The listing builds one solid part. Answer for the finished solid, in the listing's coordinates (mm). A direction names the side the tool comes from. Coordinates: 2 decimals unless noted, no trailing zeros. Write each loop counter-clockwise with the first axis right and the second up, starting at its lowest first coordinate (ties: lowest second). Pieces come first, ordered by that corner, then holes. Notation, with made-up numbers: M 42,50.25 L 58,50.25 A25 cw 58,65.25 Z; hole C 69,54 d8. An arc over 180 degrees is marked long. Answer as CSV lines item,"result". Start each with the question number.
```python
from build123d import *

# Parameters (mm, degrees)
EXTRUDE_1_DEPTH      = 90
EXTRUDE_3_DEPTH      = 45
EXTRUDE_3_DEPTH_BACK = 45
SKETCH_2_R           = 10


with BuildPart() as part:
    # Эскиз1 → Вытянуть-Тонкостенный1 (new body)
    with BuildSketch(Plane.XY):
        with BuildLine():
            Line((60, 20), (0, 20))
            ThreePointArc((0, 20), (-20, 0), (0, -20))
            Line((0, -20), (60, -20))
            Line((60, -20), (60, -10))
            Line((60, -10), (0, -10))
            ThreePointArc((0, -10), (-10, 0), (0, 10))
            Line((0, 10), (60, 10))
            Line((60, 10), (60, 20))
        make_face()
    extrude(amount=EXTRUDE_1_DEPTH)

    # Эскиз2 → Бобышка-Вытянуть3 (add, two sides: drawn at the far end of the back side and taken through both)
    with BuildSketch(Plane(origin=(0, 0, 0), x_dir=(1, 0, 0), z_dir=(0, 1, 0)).offset(-EXTRUDE_3_DEPTH_BACK)):
        with BuildLine():
            Line((-20, -25), (-20, -65))
            Line((-20, -65), (40, -65))
            ThreePointArc((40, -65), (59.396542923, -45), (40, -25))
            Line((40, -25), (-20, -25))
        make_face()
        with Locations(Location((39.387155672, -45, 0), (0, 0, 270))):
            Circle(SKETCH_2_R, mode=Mode.SUBTRACT)
    extrude(amount=EXTRUDE_3_DEPTH + EXTRUDE_3_DEPTH_BACK)


solid = part.part
```
1) The part is cut by section B-B (x = 3). Determine the outline of the cut face in (y, z), then the cut area to 3 significant figures.
2) Each of these flat-tipped pins is pushed along its axis until it touches: P1, Ø16, axis at x = 43, z = 43.5, coming from the -Y side; P2, Ø18, axis at x = 39.39, z = 45, coming from the -Y side; P3, Ø18, axis at x = 39.39, z = 45, coming from the +Y side; P4, Ø2, axis at x = 2.5, y = -24.5, coming from the +Z side. Where does it stop, or does it pass through?
3) For a pull along Z with two mould halves and no side action, classify faces 4 (the face through (39.83, -0.14, 35.01)), 5 (the face through (59.39, -32.67, 45.43)), 6 (the face through (-20, 0, 12)) as +Z half, -Z half, draft (parallel to the pull), parting line (faces both ways), or undercut.
4) Find the intervals of material crossed by line 1 (X direction, y = 35, z = 45); line 2 (Y direction, x = 23, z = 81); line 3 (Z direction, x = 10, y = 7.5), in increasing order. Write a range as from..to.
5) Which of the six approach directions +Z, -Z, +X, -X, +Y, -Y give full straight-line access (tool end or side, diameter ignored) to faces 1 (the face through (39, 10, 45)), 2 (the face through (-10, 0, 12)), 3 (the face through (30, 10, 24))?
6) The part is cut by section D-D (z = 17.5). Determine the outline of the cut face in (x, y), then the cut area to 3 significant figures.
7) The part is cut by section A-A (z = 45). Determine the outline of the cut face in (x, y), then the cut area to 3 significant figures.
8) The part is cut by section C-C (y = -3.5). Determine the outline of the cut face in (x, z).
Completed:
1,outline,"M -45,25 L -20,25 L -20,0 L -10,0 L -10,25 L 10,25 L 10,0 L 20,0 L 20,25 L 45,25 L 45,65 L 20,65 L 20,90 L 10,90 L 10,65 L -10,65 L -10,90 L -20,90 L -20,65 L -45,65 Z"
1,area,"4,600 mm²"
2,P1,"y = -45"
2,P2,"y = -20"
2,P3,"y = 20"
2,P4,"z = 65"
3,face 4,"undercut"
3,face 5,"parting line"
3,face 6,"draft"
4,line 1,"-20..29.39, 49.39..59.4"
4,line 2,"-20..-10, 10..20"
4,line 3,"25..65"
5,face 1,"none"
5,face 2,"-Z, +X"
5,face 3,"+X"
6,outline,"M 0,-20 L 60,-20 L 60,-10 L 0,-10 A10 cw 0,10 L 60,10 L 60,20 L 0,20 A20 ccw Z"
6,area,"1,670 mm²"
7,outline,"M -20,-45 L 29.39,-45 L 29.39,-20 L 49.39,-20 L 49.39,-45 L 59.4,-45 L 59.4,-20 L 60,-20 L 60,-10 L 59.4,-10 L 59.4,10 L 60,10 L 60,20 L 59.4,20 L 59.4,45 L 49.39,45 L 49.39,20 L 29.39,20 L 29.39,45 L -20,45 Z; hole M 29.39,-10 L 49.39,-10 L 49.39,10 L 29.39,10 Z"
7,area,"5,760 mm²"
8,outline,"M -20,25 L -19.69,25 L -19.69,0 L -9.37,0 L -9.37,25 L 40,25 A20.01 ccw 40,65 L -9.37,65 L -9.37,90 L -19.69,90 L -19.69,65 L -20,65 Z; hole C 39.39,45 d20"
